Part model, mm, in its own coordinate system. A direction names the side the tool comes from. Round coordinates to 2 decimals unless told otherwise and drop trailing zeros. Order: outer loops, then holes, each group sorted by start corner. A loop starts at its lowest first (then second) coordinate and runs counter-clockwise, first axis right, second up. Notation, with made-up numbers: (42, -13) -> (67, -13) arc R27 cw to (67, 20) -> close; hole circle Ø9 at (-11, 41). An arc over 180 degrees is marked (long way). Answer as a JSON object with one key per item and string values. Group by question number.
```python
from build123d import *

# Parameters (mm, degrees)
SKETCH1_R           = 2.5
BOSS_EXTRUDE1_DEPTH = 44
SKETCH2_W           = 30
SKETCH2_H           = 24
CUT_EXTRUDE1_DEPTH  = 12
FILLET1_R           = 2


with BuildPart() as part:
    # Sketch1 → Boss-Extrude1 (new body)
    with BuildSketch(Plane(origin=(0, 0, 0), x_dir=(1, 0, 0), z_dir=(0, 1, 0))):
        with BuildLine():
            Line((20, -15), (-20, -15))
            ThreePointArc((-20, -15), (-23.535533906, -13.535533906), (-25, -10))
            Line((-25, -10), (-25, 10))
            ThreePointArc((-25, 10), (-23.535533906, 13.535533906), (-20, 15))
            Line((-20, 15), (20, 15))
            ThreePointArc((20, 15), (23.535533906, 13.535533906), (25, 10))
            Line((25, 10), (25, -10))
            ThreePointArc((25, -10), (23.535533906, -13.535533906), (20, -15))
        make_face()
        with Locations((-19.5, 0)):
            Circle(SKETCH1_R, mode=Mode.SUBTRACT)
        with Locations((19.5, 0)):
            Circle(SKETCH1_R, mode=Mode.SUBTRACT)
    extrude(amount=BOSS_EXTRUDE1_DEPTH)

    # Sketch2 → Cut-Extrude1 (cut)
    with BuildSketch(Plane.ZY.offset(25)):
        with Locations((0, 22)):
            Rectangle(SKETCH2_W, SKETCH2_H)
    cut_extrude1 = extrude(amount=-CUT_EXTRUDE1_DEPTH, mode=Mode.SUBTRACT)

    # Mirror1: Cut-Extrude1 across plane
    add(cut_extrude1.mirror(Plane(origin=(0, 0, 0), x_dir=(0, 0, 1), z_dir=(1, 0, 0))), mode=Mode.SUBTRACT)

    # Fillet1
    fillet1_edges = [part.edges().sort_by_distance(p)[0] for p in [
        (-13, 34, 0),
        (-13, 10, 0),
        (13, 10, 0),
        (13, 34, 0),
    ]]
    fillet(fillet1_edges, radius=FILLET1_R)


solid = part.part
```
Q1. Which spindle directions (+Z, -Z, +X, -X, +Y, -Y) get a long thin tool onto all of the face, cutting with end or side? Do faces 5 (the flat face through (-22.3, 10, -0.2)), 6 (the cylindrical face through (13.6, 33.43, 0.21)), 7 (the cylindrical face through (24, 39, 13)). Say none if no direction does.
Q2. Band-saw the part on D-D (y = 23). List the corners of the cut face in (x, z).
Q3. Drop flat-ended pins along their axis: pin 1 Ø10 at (y, z) = (23, -1) entering from -X; pin 2 Ø4 at (x, z) = (-19.5, 0) entering from -Y; pin 3 Ø16 at (y, z) = (18.5, 6.5) entering from +X. Give the stop position or say it passes through.
Q4. Band-saw the part on B-B (z = -3.75). List the corners of the cut face in (x, y).
Q5. Wall check: line 1 (X direction, y = 38, z = 0); line 2 (Y direction, x = 22, z = 5.5); line 3 (Z direction, x = -19.5, y = 6). Give the ranges that are in metal, low to high. Write a range as [from, to].
Q6. Two-plate mould, pull along X, no slides. Class faces 1 (the flat face through (13, 22, 0)), 2 (the cylindrical face through (17, 39, 0)), 3 (the flat face through (0, 22, -15)), 4 (the cylindrical face through (-22, 39, 0)): +X half, -X half, draft (parallel to the pull), parting line (faces both ways), or undercut.
Q7. Band-saw the part on C-C (x = -19). List the corners of the cut face in (y, z).
Q8. Band-saw the part on A-A (z = 0). Count the separate pieces of the cut face and the enclosed holes in it, plus the area to 3 significant figures.
Completed:
{
 "1": {"face 5": "+Z, -Z, -X", "face 6": "+Z, -Z, +X", "face 7": "+Z, +X, +Y, -Y"},
 "2": {"outline": "(-13, -15) -> (13, -15) -> (13, 15) -> (-13, 15) -> close"},
 "3": {"pin 1": "x = -13", "pin 2": "through", "pin 3": "x = 13.68"},
 "4": {"outline": "(-25, 0) -> (25, 0) -> (25, 10) -> (15, 10) arc R2 cw to (13, 12) -> (13, 32) arc R2 cw to (15, 34) -> (25, 34) -> (25, 44) -> (-25, 44) -> (-25, 34) -> (-15, 34) arc R2 cw to (-13, 32) -> (-13, 12) arc R2 cw to (-15, 10) -> (-25, 10) -> close"},
 "5": {"line 1": "[-25, -22], [-17, 17], [22, 25]", "line 2": "[0, 10], [34, 44]", "line 3": "[-15, -2.5], [2.5, 15]"},
 "6": {"face 1": "+X half", "face 2": "undercut", "face 3": "draft", "face 4": "undercut"},
 "7": {"outline": "(0, -15) -> (10, -15) -> (10, -2.45) -> (0, -2.45) -> close; (0, 2.45) -> (10, 2.45) -> (10, 15) -> (0, 15) -> close; (34, -15) -> (44, -15) -> (44, -2.45) -> (34, -2.45) -> close; (34, 2.45) -> (44, 2.45) -> (44, 15) -> (34, 15) -> close"},
 "8": {"separate pieces": "5", "enclosed holes": "0", "area": "1,430 mm2"}
}
